Geometry: final body of the model. Coordinates: model frame, mm. A direction names the side the tool comes from. Give positions to 0.01 mm unless a question says otherwise; leave off trailing zeros. Write each loop counter-clockwise with the first axis right and the second up, starting at its lowest first coordinate (ties: lowest second). Pieces come first, ordered by that corner, then holes. Notation, with made-up numbers: M -32,61.5 L 19,61.5 A5 cw 19,69.5 Z; hole C 62,40 d8. An arc over 180 degrees is marked long. Answer as a JSON object with one key per item and string values.
from build123d import *

# Parameters (mm, degrees)
BOSS_EXTRUDE1_DEPTH      = 25
BOSS_EXTRUDE1_DEPTH_BACK = 25
SKETCH1_R                = 25
BOSS_EXTRUDE4_DEPTH      = 20
BOSS_EXTRUDE4_DEPTH_BACK = 20
SKETCH9_W                = 85
SKETCH9_H                = 20
SHELL3_START             = -18
SHELL3_DEPTH             = 36
SHELL3_START_2           = -23
SHELL3_2_OUTLINE_R       = 23
SHELL3_2_DEPTH           = 46
FILLET2_R                = 5
BOSS_EXTRUDE5_DEPTH      = 10
BOSS_EXTRUDE5_DEPTH_BACK = 10
SKETCH5_W                = 60
SKETCH5_H                = 50
BOSS_EXTRUDE3_DEPTH      = 5
CUT_EXTRUDE2_REACH       = 112.881
CHAMFER2_SIZE            = 3
SKETCH13_R               = 22.5
CUT_EXTRUDE4_DEPTH       = 1
SKETCH15_W               = 13
SKETCH15_H               = 6
CUT_EXTRUDE10_DEPTH      = 119.931868873


# Read off the part's stored shape, not the designer's step: Shell3
with BuildPart() as part:
    # Sketch1 → Boss-Extrude1 (new, two sides: drawn at the far end of the back side and taken through both)
    with BuildSketch(Plane(origin=(0, 0, 0), x_dir=(0, 0, -1), z_dir=(1, 0, 0)).offset(-BOSS_EXTRUDE1_DEPTH_BACK)):
        with Locations((-56.501901141, -5)):
            Circle(SKETCH1_R)
    extrude(amount=BOSS_EXTRUDE1_DEPTH + BOSS_EXTRUDE1_DEPTH_BACK)

    # Sketch9 → Boss-Extrude4 (add, two sides: drawn at the far end of the back side and taken through both)
    with BuildSketch(Plane(origin=(0, 0, 0), x_dir=(0, 0, -1), z_dir=(1, 0, 0)).offset(-BOSS_EXTRUDE4_DEPTH_BACK)):
        with Locations((-14.001901141, -5)):
            Rectangle(SKETCH9_W, SKETCH9_H)
    extrude(amount=BOSS_EXTRUDE4_DEPTH + BOSS_EXTRUDE4_DEPTH_BACK)

    # Shell3 outline → Shell3 (cut)
    with BuildSketch(Plane.YZ.offset(SHELL3_START)):
        with BuildLine():
            ThreePointArc((3, 34.938042488), (-5, 79.501901141), (-13, 34.938042488))
            Line((-13, 34.938042488), (-13, -26.498098859))
            Line((-13, -26.498098859), (3, -26.498098859))
            Line((3, -26.498098859), (3, 34.938042488))
        make_face()
    extrude(amount=SHELL3_DEPTH, mode=Mode.SUBTRACT)

    # Shell3 2 outline → Shell3 2 (cut)
    with BuildSketch(Plane.YZ.offset(SHELL3_START_2)):
        with Locations((-5, 56.501901141)):
            Circle(SHELL3_2_OUTLINE_R)
    extrude(amount=SHELL3_2_DEPTH, mode=Mode.SUBTRACT)

    # Fillet2
    fillet2_edges = [part.edges().sort_by_distance(p)[0] for p in [
        (0, 5, -28.498098859),
        (-20, -5, -28.498098859),
        (0, -15, -28.498098859),
        (20, -5, -28.498098859),
    ]]
    fillet(fillet2_edges, radius=FILLET2_R)

    # Sketch11 → Boss-Extrude5 (add, two sides: drawn at the far end of the back side and taken through both)
    with BuildSketch(Plane.ZY.offset(-BOSS_EXTRUDE5_DEPTH_BACK)):
        Polygon((-3.498098859, 5), (-11.271686446, 46.254104782), (-21.271686446, 46.254104782), (-23.498098859, 5), align=None)
    extrude(amount=BOSS_EXTRUDE5_DEPTH + BOSS_EXTRUDE5_DEPTH_BACK)

    # Sketch5 → Boss-Extrude3 (add)
    with BuildSketch(Plane(origin=(0, 46.254104782, 0), x_dir=(1, 0, 0), z_dir=(0, 1, 0))):
        with Locations((0, 16.271686446)):
            Rectangle(SKETCH5_W, SKETCH5_H)
    extrude(amount=BOSS_EXTRUDE3_DEPTH)

    # Sketch8 → Cut-Extrude2 (cut, up to next)
    with BuildSketch(Plane.ZY.offset(25), mode=Mode.PRIVATE) as cut_extrude2_sk1:
        Polygon((56.501901141, 12.320508076), (41.501901141, 3.660254038), (41.501901141, -13.660254038), (56.501901141, -22.320508076), (71.501901141, -13.660254038), (71.501901141, 3.660254038), align=None)
    cut_extrude2_tool1 = extrude(cut_extrude2_sk1.sketch, amount=-CUT_EXTRUDE2_REACH, mode=Mode.PRIVATE) & part.part
    add(cut_extrude2_tool1.solids().sort_by_distance((-25, -5, 56.501901))[0], mode=Mode.SUBTRACT)

    # Chamfer2
    chamfer2_edges = [part.edges().sort_by_distance(p)[0] for p in [
        (10, 25.627052391, -22.384892652),
        (10, 25.627052391, -7.384892652),
        (-10, 25.627052391, -7.384892652),
        (-10, 25.627052391, -22.384892652),
    ]]
    chamfer(chamfer2_edges, length=CHAMFER2_SIZE)

    # Sketch13 → Cut-Extrude4 (cut)
    with BuildSketch(Plane(origin=(0, 51.254104782, 0), x_dir=(1, 0, 0), z_dir=(0, 1, 0))):
        with Locations(Location((0, 16.271686446, 0), (0, 0, 270))):
            Circle(SKETCH13_R)
    extrude(amount=-CUT_EXTRUDE4_DEPTH, mode=Mode.SUBTRACT)

    # Sketch15 → Cut-Extrude10 (cut, through all)
    with BuildSketch(Plane(origin=(0, 51.254104782, 0), x_dir=(1, 0, 0), z_dir=(0, 1, 0))):
        with Locations((0, 16.271686446)):
            Rectangle(SKETCH15_W, SKETCH15_H)
    extrude(amount=-CUT_EXTRUDE10_DEPTH, mode=Mode.SUBTRACT)


solid = part.part
1) Contact query for flat-ended pins moving along their axis: P1, Ø10, axis at x = 2.5, z = 20.5, coming from the +Y side; P2, Ø6, axis at y = -10, z = -2, coming from the +X side; P3, Ø13, axis at y = -1, z = 19.5, coming from the -X side. Output: stop coordinate, or through.
Geometry check:
{"P1": "stops at y = 5", "P2": "stops at x = 20", "P3": "stops at x = -20"}
2) Cut plane C-C on z = 27.5. Return loops of the section in (x, y).
Geometry check:
{"outline": "M -20,-15 L 20,-15 L 20,5 L -20,5 Z; hole M -18,-13 L 18,-13 L 18,3 L -18,3 Z"}
3) Pull-direction query (Y, two-part tool) for faces 1 (the flat face through (0, 49, -41.272)), 2 (the flat face through (0, 51.254, -39)), 3 (the flat face through (8.521, 25.33, -8.877)); classes: pulls with the +Y half, pulls with the -Y half, needs draft (parallel to the pull), parting line crosses it, or undercut.
Geometry check:
{"face 1": "needs draft", "face 2": "pulls with the +Y half", "face 3": "undercut"}
4) Cut plane A-A on y = 10.5. Return loops of the section in (x, z).
Geometry check:
{"outline": "M -25,36.89 L 25,36.89 L 25,76.12 L -25,76.12 L -25,59.66 L -23,59.66 L -23,73.49 L 23,73.49 L 23,39.51 L -23,39.51 L -23,53.35 L -25,53.35 Z; M -10,-20.2 L -7,-23.2 L 7,-23.2 L 10,-20.2 L 10,-7.59 L 7,-4.53 L -7,-4.53 L -10,-7.59 Z; hole M -6.5,-19.27 L 6.5,-19.27 L 6.5,-13.27 L -6.5,-13.27 Z"}
5) Line query: line 1 (Y direction, x = 17.5, z = 14.5); line 2 (X direction, y = -6, z = 3.5); line 3 (Y direction, x = -9.5, z = 2). Output: solid intervals per line, ascending. Write a range as from..to.
Geometry check:
{"line 1": "y = -15..-13, 3..5", "line 2": "x = -20..-18, 18..20", "line 3": "y = -15..-13, 3..5, 46.25..50.25"}
6) Cut plane D-D on y = -5. Return loops of the section in (x, z), and give its area (3 significant figures).
Geometry check:
{"outline": "M -25,31.5 L -20,31.5 L -20,-23.5 A5 ccw -15,-28.5 L 15,-28.5 A5 ccw 20,-23.5 L 20,31.5 L 25,31.5 L 25,81.5 L -25,81.5 L -25,71.5 L -23,71.5 L -23,79.5 L 23,79.5 L 23,33.5 L 18,33.5 L 18,-26.5 L -18,-26.5 L -18,33.5 L -23,33.5 L -23,41.5 L -25,41.5 Z", "area": "553 mm2"}
7) Set-up query: faces 4 (the flat face through (-10, 21, -15)), 5 (the flat face through (0.1, 25.34, -7.33)), 6 (the cylindrical face through (0.28, 3.5, -27.07)), 7 (the flat face through (10, 21, -15)), 8 (the flat face through (-24.014, 8.051, 49.107)). Return all of +Z, -Z, +X, -X, +Y, -Y with unobstructed straight access to the full face (end or side cutting, diameter ignored); none if empty.
Geometry check:
{"face 4": "-Z, -X", "face 5": "+X, -X", "face 6": "-Z, +X, -X", "face 7": "-Z, +X", "face 8": "-X"}
